Geometry: final body of the model. Coordinates: model frame, mm. A direction names the side the tool comes from. Give positions to 0.01 mm unless a question says otherwise; leave off trailing zeros. Order: outer loops, then holes, each group sorted by start corner. A loop starts at its lowest first (then second) coordinate and runs counter-clockwise, first axis right, second up. Notation, with made-up numbers: (76.5, 37) -> (130.5, 37) arc R26 ccw to (130.5, 54) -> close; hole circle Ø11 at (8.5, -11.75). An arc over 180 degrees is marked (long way). Answer in a Markdown table with one row per item. Add a question column.
Q1. Cut plane B-B on z = 15.5. Count the separate pieces of the cut face and the enclosed holes in it, and give its area (3 significant figures).
Q2. Cut plane A-A on y = 75. Return the cut outline in (x, z).
Q3. Set-up query: faces 1 (the face through (-599.963, 4, 9)), 2 (the face through (-599.963, 90, 9)), 3 (the face through (-618.759, 47, 9)), 4 (the face through (416.037, 90, 9)). Return all of +Z, -Z, +X, -X, +Y, -Y with unobstructed straight access to the full face (end or side cutting, diameter ignored); none if empty.
Q4. Contact query for flat-ended pins moving along their axis: P1, Ø4, axis at x = 138.5, y = 12.5, coming from the -Z side; P2, Ø1, axis at y = 25, z = 4, coming from the -X side; P3, Ø8, axis at x = 428, z = 14, coming from the +Y side. Output: stop coordinate, or through.
Q5. Line query: line 1 along X through (y, z) = (8.5, 11.25); line 2 along Y through (x, z) = (391.5, 6); line 3 along Y through (x, z) = (8.5, 1.75). Output: solid intervals per line, ascending. Write a range as from..to.
Q6. Pull-direction query (X, two-part tool) for faces 5 (the face through (-99, 48, 0)), 6 (the face through (416.037, 4, 9)), 7 (the face through (-92, 48, 9.398)); classes: +X half, -X half, draft (parallel to the pull), parting line (faces both ways), or undercut.
Autodesk Inventor part; units mm, degrees
ref_plane "YZ Plane" through (0, 0, 0) normal (1, 0, 0) x (0, 1, 0)
ref_plane "XZ Plane" through (0, 0, 0) normal (0, 1, 0) x (-1, 0, 0)
ref_plane "XY Plane" through (0, 0, 0) normal (0, 0, 1) x (1, 0, 0)
sketch "Sketch1" plane through (0, 0, 0) normal (0, 0, 1) x (1, 0, 0)
  line L0 (-599.9626, 113.7827) -> (416.0374, 113.7827)
  line L1 (416.0374, -19.8213) -> (-599.9626, -19.8213)
  line L2 (-599.9626, 62.9827) -> (-618.7586, 62.9827)
  line L3 (-618.7586, 62.9827) -> (-618.7586, 30.9787)
  line L4 (-618.7586, 30.9787) -> (-599.9626, 30.9787)
  line L5 (416.0374, 62.9827) -> (434.8334, 62.9827)
  line L6 (434.8334, 62.9827) -> (434.8334, 30.9787)
  line L7 (434.8334, 30.9787) -> (416.0374, 30.9787)
  line L8 (-599.9626, -19.8213) -> (-599.9626, 30.9787)
  line L9 (-599.9626, 62.9827) -> (-599.9626, 113.7827)
  line L10 (416.0374, 113.7827) -> (416.0374, 62.9827)
  line L11 (416.0374, 30.9787) -> (416.0374, -19.8213)
  point P0 (0, 0)
  dimension "d0" = 133.604
  dimension "d1" = 1016
  dimension "d2" = 18.796
  dimension "d3" = 18.796
  dimension "d4" = 18.796
  dimension "d5" = 18.796
  dimension "d6" = 50.8
  dimension "d7" = 50.8
  dimension "d8" = 50.8
  dimension "d9" = 50.8
extrude "Extrusion1" add sketch "Sketch1" along normal blind 18.796
sketch "Sketch2" plane through (0, 0, 18.796) normal (0, 0, 1) x (1, 0, 0)
  line L0 (416.0374, 113.7827) -> (-599.9626, 113.7827)
  line L1 (-91.9626, 113.7827) -> (-91.9626, -19.8213)
  line L2 (416.0374, -19.8213) -> (-599.9626, -19.8213)
  line L3 (-101.3606, 113.7827) -> (-101.3606, -19.8213)
  line L4 (-82.5646, 113.7827) -> (-82.5646, -19.8213)
  line L5 (-101.3606, 113.7827) -> (-82.5646, 113.7827)
  line L6 (-101.3606, -19.8213) -> (-82.5646, -19.8213)
  point P0 (0, 0)
  dimension "d12" = 9.398
  dimension "d13" = 9.398
extrude "Extrusion2" cut sketch "Sketch2" against normal blind 9.398
sketch "Sketch3" plane through (0, 0, 18.796) normal (0, 0, 1) x (1, 0, 0)
  line L0 (-599.9626, 113.7827) -> (-599.9626, 62.9827)
  line L1 (-599.9626, 113.7827) -> (416.0374, 113.7827)
  point P0 (0, 0)
  point P1 (-549.1626, 88.3827)
  point P2 (-523.7626, 88.3827)
  point P3 (-498.3626, 88.3827)
  point P4 (-472.9626, 88.3827)
  point P5 (-447.5626, 88.3827)
  point P6 (-422.1626, 88.3827)
  point P7 (-396.7626, 88.3827)
  point P8 (-371.3626, 88.3827)
  point P9 (-345.9626, 88.3827)
  point P10 (-320.5626, 88.3827)
  point P11 (-295.1626, 88.3827)
  point P12 (-269.7626, 88.3827)
  point P13 (-244.3626, 88.3827)
  point P14 (-218.9626, 88.3827)
  point P15 (-193.5626, 88.3827)
  point P16 (-168.1626, 88.3827)
  point P17 (-142.7626, 88.3827)
  point P18 (-117.3626, 88.3827)
  point P19 (-91.9626, 88.3827)
  point P20 (-66.5626, 88.3827)
  point P21 (-41.1626, 88.3827)
  point P22 (-15.7626, 88.3827)
  point P23 (9.6374, 88.3827)
  point P24 (35.0374, 88.3827)
  point P25 (60.4374, 88.3827)
  point P26 (85.8374, 88.3827)
  point P27 (111.2374, 88.3827)
  point P28 (136.6374, 88.3827)
  point P29 (162.0374, 88.3827)
  point P30 (187.4374, 88.3827)
  point P31 (212.8374, 88.3827)
  point P32 (238.2374, 88.3827)
  point P33 (263.6374, 88.3827)
  point P34 (289.0374, 88.3827)
  point P35 (314.4374, 88.3827)
  point P36 (339.8374, 88.3827)
  point P37 (365.2374, 88.3827)
  point P38 (390.6374, 88.3827)
  dimension "d16" = 50.8
  dimension "d17" = 25.4
  dimension "d20" = 25.4
hole "Hole1" at (-549.1626, 88.3827, 18.796) at (-523.7626, 88.3827, 18.796) at (-498.3626, 88.3827, 18.796) at (-472.9626, 88.3827, 18.796) at (-447.5626, 88.3827, 18.796) at (-422.1626, 88.3827, 18.796) at (-396.7626, 88.3827, 18.796) at (-371.3626, 88.3827, 18.796) at (-345.9626, 88.3827, 18.796) at (-320.5626, 88.3827, 18.796) at (-295.1626, 88.3827, 18.796) at (-269.7626, 88.3827, 18.796) at (-244.3626, 88.3827, 18.796) at (-218.9626, 88.3827, 18.796) at (-193.5626, 88.3827, 18.796) at (-168.1626, 88.3827, 18.796) at (-142.7626, 88.3827, 18.796) at (-117.3626, 88.3827, 18.796) at (-91.9626, 88.3827, 18.796) at (-66.5626, 88.3827, 18.796) at (-41.1626, 88.3827, 18.796) at (-15.7626, 88.3827, 18.796) at (9.6374, 88.3827, 18.796) at (35.0374, 88.3827, 18.796) at (60.4374, 88.3827, 18.796) at (85.8374, 88.3827, 18.796) at (111.2374, 88.3827, 18.796) at (136.6374, 88.3827, 18.796) at (162.0374, 88.3827, 18.796) at (187.4374, 88.3827, 18.796) at (212.8374, 88.3827, 18.796) at (238.2374, 88.3827, 18.796) at (263.6374, 88.3827, 18.796) at (289.0374, 88.3827, 18.796) at (314.4374, 88.3827, 18.796) at (339.8374, 88.3827, 18.796) at (365.2374, 88.3827, 18.796) at (390.6374, 88.3827, 18.796) direction (0, 0, -1) diameter 6.35 end through all
sketch "Sketch4" plane through (0, 0, 18.796) normal (0, 0, 1) x (1, 0, 0)
  line L0 (-618.7586, 62.9827) -> (-599.9626, 62.9827)
  line L1 (-618.7586, 30.9787) -> (-599.9626, 30.9787)
  line L2 (416.0374, 62.9827) -> (434.8334, 62.9827)
  point P0 (0, 0)
  point P1 (416.0374, 30.9787)
hole "Hole2" at (-599.9626, 62.9827, 18.796) at (-599.9626, 30.9787, 18.796) at (416.0374, 62.9827, 18.796) at (416.0374, 30.9787, 18.796) direction (0, 0, -1) diameter 6.35 end through all
properties part number "shelf back 2" material "Wood (Birch)"
Completed:
| question | item | result |
|---|---|---|
| 1 | separate pieces | 2 |
| 1 | enclosed holes | 37 |
| 1 | area | 133,000 mm² |
| 2 | outline | (-599.96, 0) -> (416.04, 0) -> (416.04, 18.8) -> (-82.56, 18.8) -> (-82.56, 9.4) -> (-101.36, 9.4) -> (-101.36, 18.8) -> (-599.96, 18.8) -> close |
| 3 | face 1 | +Z, -Z, -X, -Y |
| 3 | face 2 | +Z, -Z, -X, +Y |
| 3 | face 3 | +Z, -Z, -X, +Y, -Y |
| 3 | face 4 | +Z, -Z, +X, +Y |
| 4 | P1 | stops at z = 0 |
| 4 | P2 | stops at x = -599.96 |
| 4 | P3 | stops at y = 62.98 |
| 5 | line 1 | x = -599.96..-101.36, -82.56..416.04 |
| 5 | line 2 | y = -19.82..85.33, 91.44..113.78 |
| 5 | line 3 | y = -19.82..85.42, 91.35..113.78 |
| 6 | face 5 | draft |
| 6 | face 6 | +X half |
| 6 | face 7 | undercut |
